The figure shows three views and two pictorial views of one solid part (mm, origin at its lowest corner). Answer the questions. Round coordinates to 2 decimals unless told otherwise and drop trailing zeros. Loops run counter-clockwise (first coordinate to the right, second up) from the corner with the lowest first, then second, coordinate; pieces in that order, holes last. Notation, with made-up numbers: (76, 62.5) -> (87, 62.5) arc R11 cw to (87, 66.5) -> close; hole circle Ø3 at (-23, 58). An arc over 180 degrees is marked (long way). Use a Markdown table: item, result. Add a question column.
Q1. For a pull along Y with two mould halves and no side action, classify the marked faces 1, 2 and 3 as released by +Y, released by -Y, zero draft, split by the parting line, or undercut.
Q2. Section B-B on x = 32 is taken. Give the vertices of the cut face in (y, z), then the cut area to 3 significant figures.
Q3. Given pin 1 Ø3 at (x, z) = (12, 6.5) entering from -Y; pin 2 Ø5 at (x, z) = (17, 2) entering from -Y, each flat-ended and moving along its own axis, determine where each tip first touches the part or whether it passes through.
Q4. Consider line 1 (X direction, y = 10, z = 3); line 2 (X direction, y = 34, z = 9); line 3 (Y direction, x = 6, z = 7.75). Determine where each line is inside the solid, lowest interval first.
Q5. Section A-A on z = 3.5 is taken. Give the vertices of the cut face in (x, y) (1 decimal), then the cut area to 3 significant figures.
Q6. Section C-C on y = 6 is taken. Give the vertices of the cut face in (x, z), then the cut area to 3 significant figures.
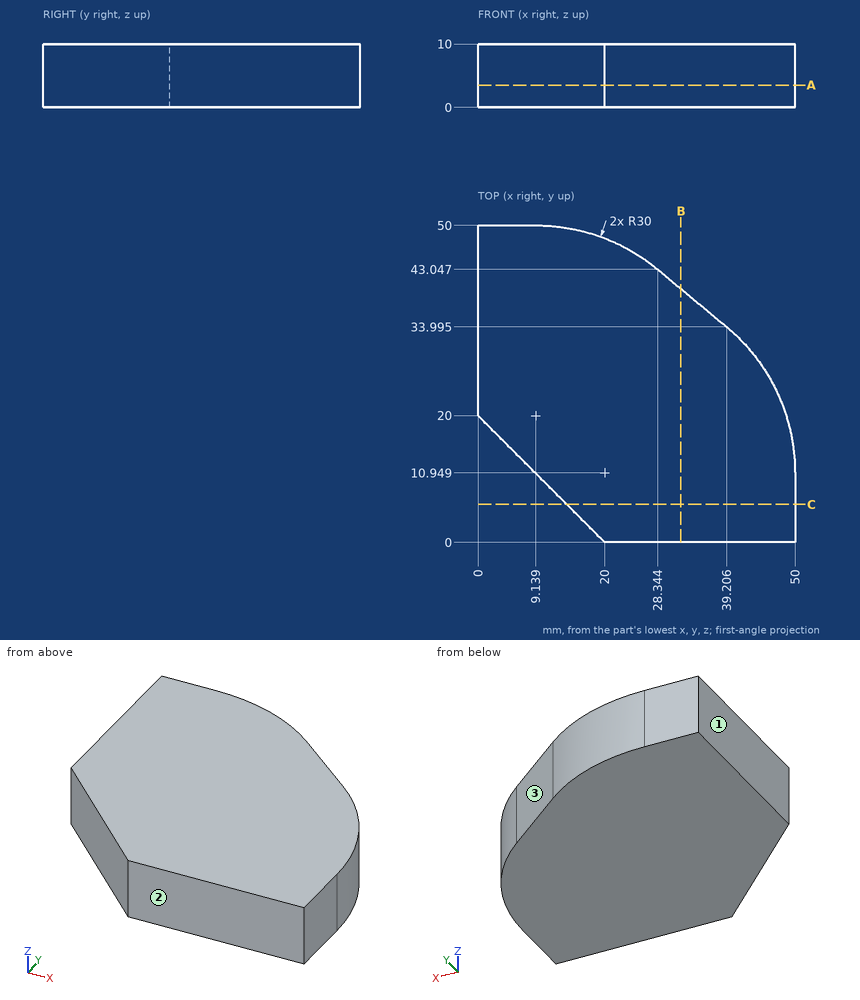
Checked values:
| question | item | result |
|---|---|---|
| 1 | face 1 | zero draft |
| 1 | face 2 | released by -Y |
| 1 | face 3 | released by +Y |
| 2 | outline | (0, 0) -> (40, 0) -> (40, 10) -> (0, 10) -> close |
| 2 | area | 400 mm2 |
| 3 | pin 1 | stops at y = 6.5 |
| 3 | pin 2 | stops at y = 0.5 |
| 4 | line 1 | x = 10 to 50 |
| 4 | line 2 | x = 0 to 39.2 |
| 4 | line 3 | y = 14 to 50 |
| 5 | outline | (0, 20) -> (20, 0) -> (50, 0) -> (50, 10.9) arc R30 ccw to (39.2, 34) -> (28.3, 43) arc R30 ccw to (9.1, 50) -> (0, 50) -> close |
| 5 | area | 1,880 mm2 |
| 6 | outline | (14, 0) -> (50, 0) -> (50, 10) -> (14, 10) -> close |
| 6 | area | 360 mm2 |
